The listing builds one solid part. Answer for the finished solid, in the listing's coordinates (mm). Coordinates: 2 decimals unless noted, no trailing zeros. Order: outer loops, then holes, each group sorted by start corner. A loop starts at its lowest first (then second) coordinate and runs counter-clockwise, first axis right, second up.
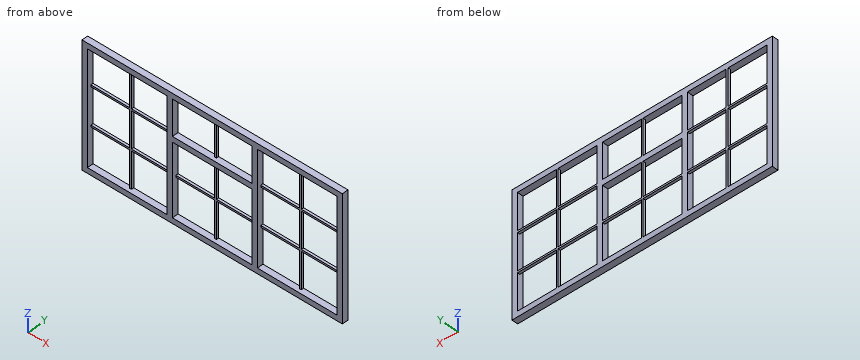
```python
from build123d import *

# Parameters (mm, degrees)
F0_W     = 2145
F0_H     = 1020
F0_W_2   = 655
F0_H_2   = 592.5
F0_H_3   = 930
F0_H_4   = 292.5
F1_DEPTH = 50
F2_W     = 320
F2_H     = 15
F2_W_2   = 15
F2_H_2   = 292.5
F3_DEPTH = 20


with BuildPart() as f1:
    # F0 (on Front) → F1 (new body)
    with BuildSketch(Plane.XZ):
        with Locations((1072.5, 510)):
            Rectangle(F0_W, F0_H)
        with Locations((1072.5, 341.25)):
            Rectangle(F0_W_2, F0_H_2, mode=Mode.SUBTRACT)
        with Locations((372.5, 510)):
            Rectangle(F0_W_2, F0_H_3, mode=Mode.SUBTRACT)
        with Locations((1772.5, 510)):
            Rectangle(F0_W_2, F0_H_3, mode=Mode.SUBTRACT)
        with Locations((1072.5, 828.75)):
            Rectangle(F0_W_2, F0_H_4, mode=Mode.SUBTRACT)
    extrude(amount=F1_DEPTH)

    # F2 (on Front) → F3 (join)
    with BuildSketch(Plane.XZ):
        Polygon((1780, 975), (1765, 975), (1765, 675), (1765, 660), (1765, 360), (1445, 360), (1445, 345), (1765, 345), (1765, 45), (1780, 45), (1780, 345), (2100, 345), (2100, 360), (1780, 360), (1780, 660), (1780, 675), align=None)
        with Locations((1605, 667.5)):
            Rectangle(F2_W, F2_H)
        with Locations((1940, 667.5)):
            Rectangle(F2_W, F2_H)
        with Locations((1072.5, 828.75)):
            Rectangle(F2_W_2, F2_H_2)
        Polygon((1080, 637.5), (1065, 637.5), (1065, 360), (745, 360), (745, 345), (1065, 345), (1065, 45), (1080, 45), (1080, 345), (1400, 345), (1400, 360), (1080, 360), align=None)
        Polygon((380, 975), (365, 975), (365, 675), (45, 675), (45, 660), (365, 660), (365, 360), (45, 360), (45, 345), (365, 345), (365, 45), (380, 45), (380, 345), (700, 345), (700, 360), (380, 360), (380, 660), (700, 660), (700, 675), (380, 675), align=None)
    extrude(amount=F3_DEPTH)


solid = f1.part
```
(1) Find section C-C (y = -36). Write down the section's boundary in (x, z).
(2) Find section A-A (z = 549.5). Write down the section's boundary in (x, y), and give its area (3 significant figures).
(3) Find section D-D (x = 568.5). Write down the section's boundary in (y, z), and give its area (3 significant figures).
(4) Consider line 1 (X direction, y = -45.5, z = 630); line 2 (Z direction, x = 390.5, y = -8); line 3 (X direction, y = -42, z = 669). Determine where each line is inside the solid, lowest interval first.
(5) This flat-tipped pin is pushed along its axis until it touches: pin 1 Ø6 at (x, z) = (1575, 341) entering from +Y. Where does it stop, or does it pass through?
(6) Find section B-B (x = 1188). Write down the section's boundary in (y, z), and give its area (3 significant figures).
Findings below:
1. outline: (0, 0) - (2145, 0) - (2145, 1020) - (0, 1020) - close; hole (45, 45) - (700, 45) - (700, 975) - (45, 975) - close; hole (745, 45) - (1400, 45) - (1400, 637.5) - (745, 637.5) - close; hole (745, 682.5) - (1400, 682.5) - (1400, 975) - (745, 975) - close; hole (1445, 45) - (2100, 45) - (2100, 975) - (1445, 975) - close
2. outline: (0, -50) - (45, -50) - (45, 0) - (0, 0) - close; (365, -20) - (380, -20) - (380, 0) - (365, 0) - close; (700, -50) - (745, -50) - (745, 0) - (700, 0) - close; (1065, -20) - (1080, -20) - (1080, 0) - (1065, 0) - close; (1400, -50) - (1445, -50) - (1445, 0) - (1400, 0) - close; (1765, -20) - (1780, -20) - (1780, 0) - (1765, 0) - close; (2100, -50) - (2145, -50) - (2145, 0) - (2100, 0) - close
2. area: 9,900 mm2
3. outline: (-50, 0) - (0, 0) - (0, 45) - (-50, 45) - close; (-50, 975) - (0, 975) - (0, 1020) - (-50, 1020) - close; (-20, 345) - (0, 345) - (0, 360) - (-20, 360) - close; (-20, 660) - (0, 660) - (0, 675) - (-20, 675) - close
3. area: 5,100 mm2
4. line 1: x = 0 to 45, 700 to 745, 1400 to 1445, 2100 to 2145
4. line 2: z = 0 to 45, 345 to 360, 660 to 675, 975 to 1020
4. line 3: x = 0 to 45, 700 to 1445, 2100 to 2145
5. pin 1: passes through
6. outline: (-50, 0) - (0, 0) - (0, 45) - (-50, 45) - close; (-50, 637.5) - (0, 637.5) - (0, 682.5) - (-50, 682.5) - close; (-50, 975) - (0, 975) - (0, 1020) - (-50, 1020) - close; (-20, 345) - (0, 345) - (0, 360) - (-20, 360) - close
6. area: 7,050 mm2
